Design review of the part built by this model. Coordinates are the model's own, in mm. Face numbers are marked on the shaded views. A direction names the side the tool comes from. Round coordinates to 2 decimals unless told otherwise and drop trailing zeros. Use a Markdown table: item, result. Add a question column.
(1) Machinability: for the marked faces 5 and 6, which of the approach directions +Z, -Z, +X, -X, +Y, -Y give a long, thin tool a straight path to every point of the face, cutting with its end or side? Answer none if there is none.
(2) The part is to be moulded in two halves that separate along Z. For the marked faces 1, 2, 3 and 4, say which applies: released by +Z, released by -Z, zero draft, split by the parting line, or undercut.
(3) To check wall thickness, follow probe 1 along Z at (x, y) = (0, 2.5); probe 2 along Z at (x, y) = (0, -7.75). State the ranges of each line that lie inside material, in increasing order. Write a range as from..to.
(4) For pin 1 (4 mm diameter, centred on y = 2.5, z = 2.5, fed in from +X); pin 2 (2 mm diameter, centred on x = 4, y = -7.5, fed in from -Z); pin 3 (1.5 mm diameter, centred on x = 1.5, z = -9, fed in from -Y); pin 4 (1 mm diameter, centred on x = 3, z = -3.5, fed in from -Y), all flat-tipped, find the tip position at first contact; note any pin that passes through.
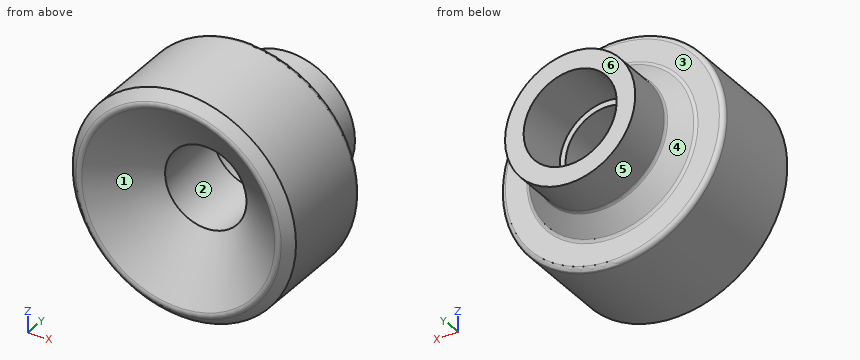
```python
from build123d import *

# Parameters (mm, degrees)
CHAMFER1_SIZE                   = 1.905
FILLET1_R                       = 0.635
F_7_16_0_4375_DOWEL_HOLE1_D     = 11.1125
F_7_16_0_4375_DOWEL_HOLE1_DEPTH = 11.938
F_7_16_0_4375_DOWEL_HOLE1_TIP   = 3.338531814


with BuildPart() as part:
    # Sketch1 → Revolve1 (revolve)
    with BuildSketch(Plane.XY):
        Polygon((0, 0), (6.35, 0), (6.35, 7.62), (8.89, 7.62), (8.89, 1.27), (11.43, -1.27), (15.24, -1.27), (15.24, -16.51), (13.97, -16.51), (0, -5.837068859), align=None)
    revolve(axis=Axis((0, -1033.02, 0), (0, 1, 0)))

    # Chamfer1
    # the kernel refuses this chamfer: 1.905 mm, written as the material it takes off along each edge
    with BuildSketch(Plane(origin=(0, -16.51, 0), x_dir=(1, 0, 0), z_dir=(0, 0, 1))) as chamfer1_piece_1:
        Polygon((15.24, CHAMFER1_SIZE), (15.24 - CHAMFER1_SIZE, 0), (15.24, 0), align=None)
    revolve(axis=Axis((0, -16.51, 0), (0, 1, 0)), mode=Mode.SUBTRACT)

    # Fillet1
    fillet1_edges = [part.edges().sort_by_distance(p)[0] for p in [
        (-13.610020501, -16.234979499, 0),
        (-15.24, -1.27, 0),
        (-11.43, -1.27, 0),
        (-8.89, 1.27, 0),
    ]]
    fillet(fillet1_edges, radius=FILLET1_R)

    # 7/16 (0.4375) Dowel Hole1
    with Locations(Plane(origin=(0, 0, 0), x_dir=(1, 0, 0), z_dir=(0, 1, 0))):
        with Locations((0, 0)):
            Hole(F_7_16_0_4375_DOWEL_HOLE1_D / 2, depth=F_7_16_0_4375_DOWEL_HOLE1_DEPTH)
            with Locations((0, 0, -(F_7_16_0_4375_DOWEL_HOLE1_DEPTH + F_7_16_0_4375_DOWEL_HOLE1_TIP / 2))):  # 118° drill point
                Cone(0, F_7_16_0_4375_DOWEL_HOLE1_D / 2, F_7_16_0_4375_DOWEL_HOLE1_TIP, mode=Mode.SUBTRACT)


solid = part.part
```
Verdict:
| question | item | result |
|---|---|---|
| 1 | face 5 | +Y |
| 1 | face 6 | +Z, -Z, +X, -X, +Y |
| 2 | face 1 | undercut |
| 2 | face 2 | undercut |
| 2 | face 3 | zero draft |
| 2 | face 4 | split by the parting line |
| 3 | probe 1 | z = -8.89..-6.35, 6.35..8.89 |
| 3 | probe 2 | z = -15.24..-5.56, 5.56..15.24 |
| 4 | pin 1 | stops at x = 9.39 |
| 4 | pin 2 | stops at z = -14.94 |
| 4 | pin 3 | stops at y = -13.38 |
| 4 | pin 4 | passes through |
